Geometry check sheet. Reference: the model listing, model coordinates, mm. A direction names the side the tool comes from. Give positions to 0.01 mm unless a question says otherwise; leave off trailing zeros. Write each loop counter-clockwise with the first axis right and the second up, starting at its lowest first coordinate (ties: lowest second). Pieces come first, ordered by that corner, then holes.
(1) Tool access check on faces 5 (the flat face through (-1, 62.23, 2)), 6 (the flat face through (-2.794, 61, 0)). Record the directions out of +Z, -Z, +X, -X, +Y, -Y that give a thin tool (end or side, any length) a straight path to the whole face; none if there is none.
(2) Mould release check, pull along Z, two halves, no side actions. Record for faces 1 (the flat face through (0, 50.546, 0)), 2 (the cylindrical face through (0.652, 56.118, 1.572)), 3 (the flat face through (2.794, 61, 0)), 4 (the cylindrical face through (-0.69, 30.68, -3.1)): +Z half, -Z half, draft (parallel to the pull), parting line (faces both ways), or undercut.
(3) Depth check by flat-ended pin: P1, Ø1.5, axis at y = 48.5, z = 2.5, coming from the +X side; P2, Ø0.9, axis at y = 60.5, z = -0.5, coming from the +X side; P3, Ø1.7, axis at x = -0.5, z = -0.5, coming from the +Y side. Enter the tip coordinate at first touch or a pass-through.
(4) Cross-section at A-A (x = 0). Record the boundary of the cut face in (y, z) (3 decimals), and give its area (3 significant figures).
(5) Thickness scan on line 1 along X through (y, z) = (59.5, 0); line 2 along X through (y, z) = (57, 0) (3 decimals). Record the ranges inside material, lowest first.
(6) Cross-section at B-B (y = 51.5). Record the boundary of the cut face in (x, z) (3 decimals), and give its area (3 significant figures).
(7) Cross-section at C-C (y = 26). Record the boundary of the cut face in (x, z) (3 decimals).
Autodesk Inventor part; units mm, degrees
ref_plane "b11_XY" through (0, 0, 0) normal (0, 1, 0) x (1, 0, 0)
ref_plane "b11_YZ" through (0, 0, 0) normal (1, 0, 0) x (0, 0, -1)
ref_plane "b11_ZX" through (0, 0, 0) normal (0, 0, -1) x (0, 1, 0)
sketch "Sketch_1" plane through (0, 0, 0) normal (0, 0, 1) x (1, 0, 0)
  line L0 (0, 0) -> (0, 62.23)
  line L1 (0, 62.23) -> (3.175, 62.23)
  line L2 (3.175, 62.23) -> (3.175, 0)
  line L3 (3.175, 0) -> (0, 0)
  line L4 (0, 0) -> (0, 62.23)
revolve "Revolution1" add sketch "Sketch_1" angle 360 about axis through (0, 0, 0) along (0, -1, 0)
sketch "Sketch2" plane through (0, 62.23, 0) normal (0, 1, 0) x (1, 0, 0)
  point P0 (0, 0)
hole "Hole1" at (0, 62.23, 0) direction (0, -1, 0) diameter 3.4036 depth 11.684 countersink diameter 4.1656 countersink angle 90
sketch "Sketch_29" plane through (0, 62.23, 0) normal (0, 1, 0) x (1, 0, 0)
  line L0 (-5.588, 12.7) -> (-5.588, -12.7)
  line L1 (-5.588, -12.7) -> (5.588, -12.7)
  line L2 (5.588, -12.7) -> (5.588, 12.7)
  line L3 (5.588, 12.7) -> (-5.588, 12.7)
  line L4 (-2.794, 6.35) -> (-2.794, -6.35)
  line L5 (-2.794, -6.35) -> (2.794, -6.35)
  line L6 (2.794, -6.35) -> (2.794, 6.35)
  line L7 (2.794, 6.35) -> (-2.794, 6.35)
extrude "Extrusion1" cut sketch "Sketch_29" against normal blind 3.302
ref_plane "b11_XY" through (0, 0, 0) normal (0, 1, 0) x (1, 0, 0)
ref_plane "b11_YZ" through (0, 0, 0) normal (1, 0, 0) x (0, 0, -1)
ref_plane "b11_ZX" through (0, 0, 0) normal (0, 0, -1) x (0, 1, 0)
ref_plane "b2_XY" through (0, 62.23, 0) normal (0, 1, 0) x (1, 0, 0)
ref_plane "b2_YZ" through (0, 62.23, 0) normal (1, 0, 0) x (0, 0, -1)
ref_plane "b2_ZX" through (0, 62.23, 0) normal (0, 0, -1) x (0, 1, 0)
ref_plane "e1_XY" through (0, 62.23, -2.0828) normal (1, 0, 0) x (0, 0, -1)
ref_plane "e1_YZ" through (0, 62.23, -2.0828) normal (0, 0, -1) x (0, 1, 0)
ref_plane "e1_ZX" through (0, 62.23, -2.0828) normal (0, 1, 0) x (1, 0, 0)
ref_plane "e2_XY" through (0, 62.23, 2.0828) normal (1, 0, 0) x (0, 0, -1)
ref_plane "e2_YZ" through (0, 62.23, 2.0828) normal (0, 0, -1) x (0, 1, 0)
ref_plane "e2_ZX" through (0, 62.23, 2.0828) normal (0, 1, 0) x (1, 0, 0)
ref_plane "f1_XY" through (0, 62.23, 3.175) normal (1, 0, 0) x (0, 0, -1)
ref_plane "f1_YZ" through (0, 62.23, 3.175) normal (0, 0, -1) x (0, 1, 0)
ref_plane "f1_ZX" through (0, 62.23, 3.175) normal (0, 1, 0) x (1, 0, 0)
ref_plane "f2_XY" through (0, 62.23, -3.175) normal (1, 0, 0) x (0, 0, -1)
ref_plane "f2_YZ" through (0, 62.23, -3.175) normal (0, 0, -1) x (0, 1, 0)
ref_plane "f2_ZX" through (0, 62.23, -3.175) normal (0, 1, 0) x (1, 0, 0)
ref_plane "h1_XY" through (-2.794, 62.23, 0) normal (0, 1, 0) x (1, 0, 0)
ref_plane "h1_YZ" through (-2.794, 62.23, 0) normal (1, 0, 0) x (0, 0, -1)
ref_plane "h1_ZX" through (-2.794, 62.23, 0) normal (0, 0, -1) x (0, 1, 0)
ref_plane "h2_XY" through (2.794, 62.23, 0) normal (0, 1, 0) x (1, 0, 0)
ref_plane "h2_YZ" through (2.794, 62.23, 0) normal (1, 0, 0) x (0, 0, -1)
ref_plane "h2_ZX" through (2.794, 62.23, 0) normal (0, 0, -1) x (0, 1, 0)
ref_plane "rod_XY" through (0, 62.23, 0) normal (0, 1, 0) x (1, 0, 0)
ref_plane "rod_YZ" through (0, 62.23, 0) normal (1, 0, 0) x (0, 0, -1)
ref_plane "rod_ZX" through (0, 62.23, 0) normal (0, 0, -1) x (0, 1, 0)
ref_plane "rod_to_part_XY" through (0, 0, 0) normal (0, 1, 0) x (1, 0, 0)
ref_plane "rod_to_part_YZ" through (0, 0, 0) normal (1, 0, 0) x (0, 0, -1)
ref_plane "rod_to_part_ZX" through (0, 0, 0) normal (0, 0, -1) x (0, 1, 0)
ref_plane "to_rod_pivot_XY" through (0, 62.23, 0) normal (0, 1, 0) x (1, 0, 0)
ref_plane "to_rod_pivot_YZ" through (0, 62.23, 0) normal (1, 0, 0) x (0, 0, -1)
ref_plane "to_rod_pivot_ZX" through (0, 62.23, 0) normal (0, 0, -1) x (0, 1, 0)
ref_plane "to_rod_pivot1_XY" through (0, 0, 0) normal (0, 1, 0) x (1, 0, 0)
ref_plane "to_rod_pivot1_YZ" through (0, 0, 0) normal (1, 0, 0) x (0, 0, -1)
ref_plane "to_rod_pivot1_ZX" through (0, 0, 0) normal (0, 0, -1) x (0, 1, 0)
properties part number "022.452.45-FO1_BM_rod" material "Steel"
Reply:
1. face 5: +Z, -Z, +X, -X, +Y
1. face 6: +Z, -Z, -X, +Y
2. face 1: undercut
2. face 2: undercut
2. face 3: draft
2. face 4: parting line
3. P1: stops at x = 2.65
3. P2: stops at x = 2.79
3. P3: stops at y = 50.55
4. outline: (0, -3.175) - (62.23, -3.175) - (62.23, -2.083) - (61.849, -1.702) - (50.546, -1.702) - (50.546, 1.702) - (61.849, 1.702) - (62.23, 2.083) - (62.23, 3.175) - (0, 3.175) - close
4. area: 355 mm2
5. line 1: x = -2.79 to -1.7, 1.7 to 2.79
5. line 2: x = -3.175 to -1.702, 1.702 to 3.175
6. outline: circle Ø6.35 at (0, 0); hole circle Ø3.404 at (0, 0)
6. area: 22.6 mm2
7. outline: circle Ø6.35 at (0, 0)
